Design review of the part built by this model. Coordinates are the model's own, in mm. A direction names the side the tool comes from. Coordinates: 2 decimals unless noted, no trailing zeros. Loops run counter-clockwise (first coordinate to the right, second up) from the corner with the lowest first, then second, coordinate; pieces in that order, holes last. Notation, with made-up numbers: (72.25, 48.5) - (93.25, 48.5) arc R16 ccw to (93.25, 74.5) - close; hole circle Ø7 at (45, 37). An arc over 180 degrees is marked (long way). Answer in a Markdown table with one row per item. Add a question column.
(1) The part is to be moulded in two halves that separate along Z. For faces 4 (the face through (-3, 10, 45.5)), 5 (the face through (-3, 10, 42.5)), 6 (the face through (108.5, 27, 23)), say which applies: released by +Z, released by -Z, zero draft, split by the parting line, or undercut.
(2) We need section C-C, the plane x = -48. Write out the cut boundary in (y, z).
(3) Clearance check with flat-ended pins moving along their axes: pin 1 (7.5 mm diameter, centred on x = 107.5, y = 14.5, fed in from +Z); pin 2 (15 mm diameter, centred on x = 15, y = 10, fed in from -Z); pin 3 (0.8 mm diameter, centred on x = 103.5, y = -1, fed in from +Z). State where each tip first meets the part, or that it passes through.
(4) We need section D-D, the plane z = -21.5. Write out the cut boundary in (x, y), plus the area to 3 significant figures.
(5) To check wall thickness, follow L1, parallel to Z at x = 110.2, y = 29; L2, parallel to Z at x = 86, y = 13; L3, parallel to Z at x = 109.15, y = 13.5. State the ranges of each line that lie inside material, in increasing order. Write a range as [from, to].
(6) For faces 1 (the face through (-3, 0, -1)), 2 (the face through (0, 19.5, 57)), 3 (the face through (104.5, -1, -35)), list the 3-axis set-ups (+Z, -Z, +X, -X, +Y, -Y) from which the entire face can be reached by the end or side of a thin tool; tool diameter is ignored.
(7) We need section B-B, the plane y = 13.5. Write out the cut boundary in (x, z).
(8) We need section A-A, the plane z = 22.5. Write out the cut boundary in (x, y).
from build123d import *

# Parameters (mm, degrees)
BASE_FLANGE1_DEPTH            = 3
EDGE_FLANGE1_STRIP_W          = 20
EDGE_FLANGE1_STRIP_H          = 3
EDGE_FLANGE1_STRIP_CUT_DEPTH  = 40
EDGE_FLANGE1_RELIEF_W         = 21.5
EDGE_FLANGE1_RELIEF_H         = 1.5
EDGE_FLANGE1_RELIEF_CUT_DEPTH = 3
EDGE_FLANGE1_DEPTH            = 40
SKETCH10_R                    = 1.75
SKETCH10_R_2                  = 6
CUT_EXTRUDE1_DEPTH            = 226.814636372
EDGE_FLANGE2_STRIP_W          = 18
EDGE_FLANGE2_STRIP_H          = 3
EDGE_FLANGE2_STRIP_CUT_DEPTH  = 212
EDGE_FLANGE2_DEPTH            = 212
EDGE_FLANGE3_STRIP_W          = 18
EDGE_FLANGE3_STRIP_H          = 3
EDGE_FLANGE3_STRIP_CUT_DEPTH  = 212
EDGE_FLANGE3_DEPTH            = 212
MIRROR1_START                 = -107.5
MIRROR1_DEPTH                 = 213.5
MIRROR1_START_2               = 104.5
MIRROR1_2_DEPTH               = 1.5
MIRROR1_3_DEPTH               = 212
TAB1_DEPTH                    = 3
CUT_EXTRUDE2_DEPTH            = 10


# Read off the part's stored shape, not the designer's step: Mirror1
# Sheet-metal steps are written as plain solids
with BuildPart() as part:
    # Sketch1 → Base-Flange1 (new body)
    with BuildSketch(Plane(origin=(0, 0, 0), x_dir=(1, 0, 0), z_dir=(0, 1, 0))):
        Polygon((-107.5, -42.5), (108.5, -42.5), (108.5, -2.5), (107.5, -2.5), (107.5, 42.5), (-107.5, 42.5), align=None)
    extrude(amount=-BASE_FLANGE1_DEPTH)

    # Edge-Flange1 strip (across the edge) → Edge-Flange1 strip cut (cut)
    with BuildSketch(Plane(origin=(108.5, 0, 42.5), x_dir=(-1, 0, 0), z_dir=(0, 0, -1))):
        with Locations((-6, -1.5)):
            Rectangle(EDGE_FLANGE1_STRIP_W, EDGE_FLANGE1_STRIP_H)
    extrude(amount=EDGE_FLANGE1_STRIP_CUT_DEPTH, mode=Mode.SUBTRACT)

    # Edge-Flange1 relief (on the sheet) → Edge-Flange1 relief cut (cut)
    with BuildSketch(Plane(origin=(104.5, 0, 42.5), x_dir=(-1, 0, 0), z_dir=(0, 1, 0))):
        with Locations((-9.25, -40.75)):
            Rectangle(EDGE_FLANGE1_RELIEF_W, EDGE_FLANGE1_RELIEF_H)
    extrude(amount=-EDGE_FLANGE1_RELIEF_CUT_DEPTH, mode=Mode.SUBTRACT)

    # Edge-Flange1 section (across the edge) → Edge-Flange1 (add)
    with BuildSketch(Plane(origin=(108.5, 0, 42.5), x_dir=(-1, 0, 0), z_dir=(0, 0, -1))):
        with BuildLine():
            Line((-3, 4), (-3, 35))
            Line((-3, 35), (0, 35))
            Line((0, 35), (0, 4))
            ThreePointArc((0, 4), (1.171572875, 1.171572875), (4, 0))
            Line((4, 0), (4, -3))
            ThreePointArc((4, -3), (-0.949747468, -0.949747468), (-3, 4))
        make_face()
    extrude(amount=EDGE_FLANGE1_DEPTH)

    # Sketch10 → Cut-Extrude1 (cut, through all)
    with BuildSketch(Plane(origin=(111.5, 0, 0), x_dir=(0, 0, -1), z_dir=(1, 0, 0))):
        with Locations(Location((-38, 29, 0), (0, 0, 90))):
            Circle(SKETCH10_R)
        with Locations(Location((-7, 29, 0), (0, 0, 90))):
            Circle(SKETCH10_R)
        with Locations(Location((-22.5, 13.5, 0), (0, 0, 90))):
            Circle(SKETCH10_R_2)
    extrude(amount=-CUT_EXTRUDE1_DEPTH, mode=Mode.SUBTRACT)

    # Edge-Flange2 strip (across the edge) → Edge-Flange2 strip cut (cut)
    with BuildSketch(Plane(origin=(-107.5, 0, 42.5), x_dir=(0, 0, -1), z_dir=(1, 0, 0))):
        with Locations((-6, -1.5)):
            Rectangle(EDGE_FLANGE2_STRIP_W, EDGE_FLANGE2_STRIP_H)
    extrude(amount=EDGE_FLANGE2_STRIP_CUT_DEPTH, mode=Mode.SUBTRACT)

    # Edge-Flange2 section (across the edge) → Edge-Flange2 (add)
    with BuildSketch(Plane(origin=(-107.5, 0, 42.5), x_dir=(0, 0, -1), z_dir=(1, 0, 0))):
        with BuildLine():
            Line((-3, 3), (-3, 19.5))
            Line((-3, 19.5), (0, 19.5))
            Line((0, 19.5), (0, 3))
            ThreePointArc((0, 3), (0.878679656, 0.878679656), (3, 0))
            Line((3, 0), (3, -3))
            ThreePointArc((3, -3), (-1.242640687, -1.242640687), (-3, 3))
        make_face()
    extrude(amount=EDGE_FLANGE2_DEPTH)

    # Edge-Flange3 strip (across the edge) → Edge-Flange3 strip cut (cut)
    with BuildSketch(Plane(origin=(104.5, 19.5, 45.5), x_dir=(0, -1, 0), z_dir=(-1, 0, 0))):
        with Locations((-6, -1.5)):
            Rectangle(EDGE_FLANGE3_STRIP_W, EDGE_FLANGE3_STRIP_H)
    extrude(amount=EDGE_FLANGE3_STRIP_CUT_DEPTH, mode=Mode.SUBTRACT)

    # Edge-Flange3 section (across the edge) → Edge-Flange3 (add)
    with BuildSketch(Plane(origin=(104.5, 19.5, 45.5), x_dir=(0, -1, 0), z_dir=(-1, 0, 0))):
        with BuildLine():
            Line((-3, 3), (-3, 20))
            Line((-3, 20), (0, 20))
            Line((0, 20), (0, 3))
            ThreePointArc((0, 3), (0.878679656, 0.878679656), (3, 0))
            Line((3, 0), (3, -3))
            ThreePointArc((3, -3), (-1.242640687, -1.242640687), (-3, 3))
        make_face()
    extrude(amount=EDGE_FLANGE3_DEPTH)

    # Mirror1 outline → Mirror1 (cut)
    with BuildSketch(Plane.YZ.offset(MIRROR1_START)):
        with BuildLine():
            Line((-3, -42.5), (-2.196152423, -42.5))
            ThreePointArc((-2.196152423, -42.5), (-2.795554958, -41.052914271), (-3, -39.5))
            Line((-3, -39.5), (-3, -42.5))
        make_face()
    extrude(amount=MIRROR1_DEPTH, mode=Mode.SUBTRACT)

    # Mirror1 2 outline → Mirror1 2 (cut)
    with BuildSketch(Plane.YZ.offset(MIRROR1_START_2)):
        with BuildLine():
            ThreePointArc((-3, -39.5), (-2.795554958, -41.052914271), (-2.196152423, -42.5))
            Line((-2.196152423, -42.5), (0, -42.5))
            Line((0, -42.5), (0, -38))
            Line((0, -38), (-3, -38))
            Line((-3, -38), (-3, -39.5))
        make_face()
    extrude(amount=MIRROR1_2_DEPTH, mode=Mode.SUBTRACT)

    # Mirror1 3 outline → Mirror1 3 (add)
    with BuildSketch(Plane.YZ.offset(MIRROR1_START)):
        with BuildLine():
            Line((3, -45.5), (16.5, -45.5))
            ThreePointArc((16.5, -45.5), (18.621320344, -46.378679656), (19.5, -48.5))
            Line((19.5, -48.5), (19.5, -65.5))
            Line((19.5, -65.5), (22.5, -65.5))
            Line((22.5, -65.5), (22.5, -48.5))
            ThreePointArc((22.5, -48.5), (20.742640687, -44.257359313), (16.5, -42.5))
            Line((16.5, -42.5), (3, -42.5))
            ThreePointArc((3, -42.5), (0.878679656, -41.621320344), (0, -39.5))
            Line((0, -39.5), (0, -42.5))
            Line((0, -42.5), (-2.196152423, -42.5))
            ThreePointArc((-2.196152423, -42.5), (0, -44.696152423), (3, -45.5))
        make_face()
    extrude(amount=MIRROR1_3_DEPTH)

    # Sketch18 → Tab1 (add)
    with BuildSketch(Plane(origin=(111.5, 0, 0), x_dir=(0, 0, -1), z_dir=(1, 0, 0))):
        with BuildLine():
            Line((-42.5, 35), (-2.5, 35))
            Line((-2.5, 35), (-2.5, 40))
            ThreePointArc((-2.5, 40), (-5.428932188, 47.071067812), (-12.5, 50))
            Line((-12.5, 50), (-32.5, 50))
            ThreePointArc((-32.5, 50), (-39.571067812, 47.071067812), (-42.5, 40))
            Line((-42.5, 40), (-42.5, 35))
        make_face()
    extrude(amount=-TAB1_DEPTH)

    # Sketch19 → Cut-Extrude2 (cut)
    with BuildSketch(Plane(origin=(0, 0, 0), x_dir=(1, 0, 0), z_dir=(0, 1, 0))):
        Polygon((107.5, -1), (107.5, 42.5), (106, 42.5), (104.5, 38), (104.5, -1), align=None)
    extrude(amount=-CUT_EXTRUDE2_DEPTH, mode=Mode.SUBTRACT)


solid = part.part
Responses:
| question | item | result |
|---|---|---|
| 1 | face 4 | released by +Z |
| 1 | face 5 | undercut |
| 1 | face 6 | zero draft |
| 2 | outline | (-3, -39.5) arc R6 ccw to (3, -45.5) - (16.5, -45.5) arc R3 cw to (19.5, -48.5) - (19.5, -65.5) - (22.5, -65.5) - (22.5, -48.5) arc R6 ccw to (16.5, -42.5) - (3, -42.5) arc R3 cw to (0, -39.5) - (0, 39.5) arc R3 cw to (3, 42.5) - (16.5, 42.5) arc R6 ccw to (22.5, 48.5) - (22.5, 65.5) - (19.5, 65.5) - (19.5, 48.5) arc R3 cw to (16.5, 45.5) - (3, 45.5) arc R6 ccw to (-3, 39.5) - close |
| 3 | pin 1 | stops at z = 45.51 |
| 3 | pin 2 | stops at z = -45.67 |
| 3 | pin 3 | stops at z = 44.3 |
| 4 | outline | (-107.5, -3) - (104.5, -3) - (104.5, 0) - (-107.5, 0) - close |
| 4 | area | 636 mm2 |
| 5 | L1 | z = [2.5, 5.25], [8.75, 36.25], [39.75, 42.5] |
| 5 | L2 | z = [-45.5, -42.5], [42.5, 45.5] |
| 5 | L3 | z = [2.5, 16.5], [28.5, 42.5] |
| 6 | face 1 | -X, +Y |
| 6 | face 2 | +Z, +X, -X, -Y |
| 6 | face 3 | -Z, +X, +Y, -Y |
| 7 | outline | (-107.5, -45.5) - (104.5, -45.5) - (104.5, -42.5) - (-107.5, -42.5) - close; (-107.5, 42.5) - (104.5, 42.5) - (104.5, 45.5) - (-107.5, 45.5) - close; (108.5, 2.5) - (111.5, 2.5) - (111.5, 16.5) - (108.5, 16.5) - close; (108.5, 28.5) - (111.5, 28.5) - (111.5, 42.5) - (108.5, 42.5) - close |
| 8 | outline | (-107.5, -3) - (104.5, -3) arc R7 ccw to (111.5, 4) - (111.5, 7.5) - (108.5, 7.5) - (108.5, 4) arc R4 cw to (104.5, 0) - (-107.5, 0) - close; (108.5, 19.5) - (111.5, 19.5) - (111.5, 50) - (108.5, 50) - close |
